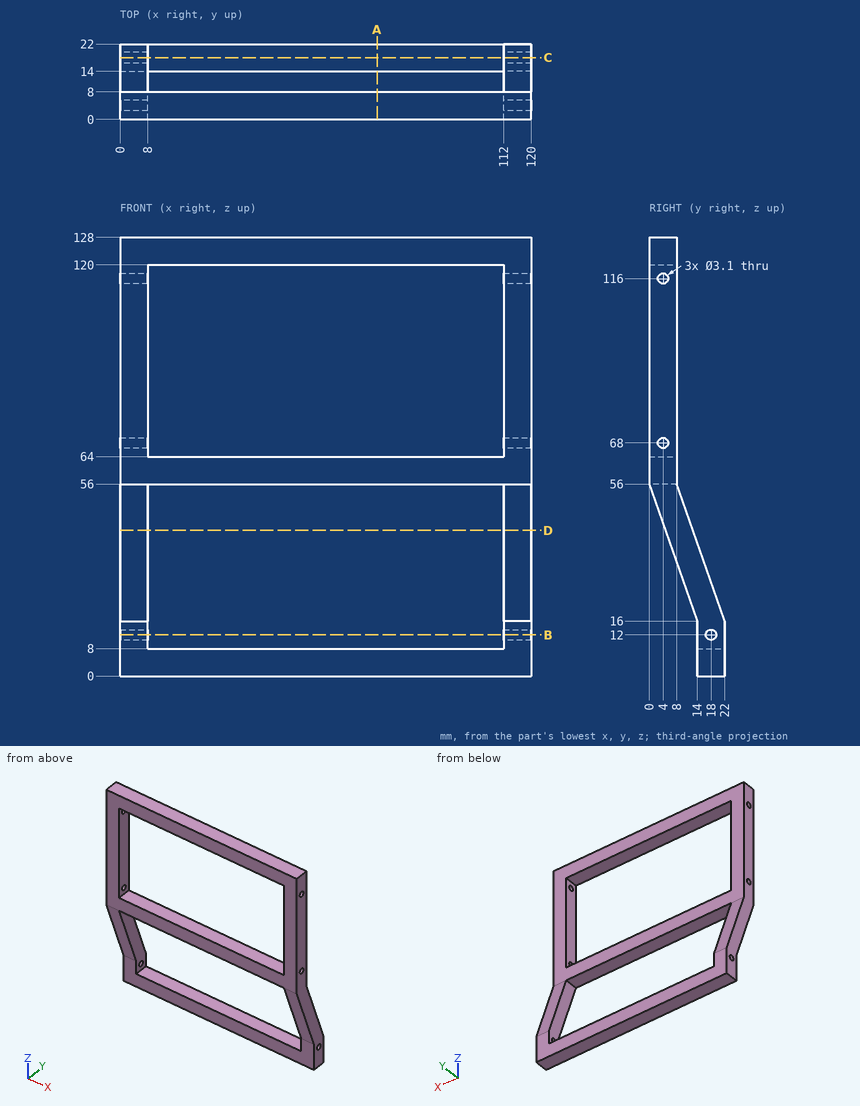
Could you check a few things on this drawing? It's one solid part, dimensions in mm from its lowest x, y, z. Round coordinates to 2 decimals unless told otherwise and drop trailing zeros. Write each loop counter-clockwise with the first axis right and the second up, starting at its lowest first coordinate (ties: lowest second). Pieces come first, ordered by that corner, then holes. Notation, with made-up numbers: (71, 13.5) -> (119, 13.5) arc R5 cw to (119, 17.5) -> close; hole circle Ø6 at (-21.75, 63). An arc over 180 degrees is marked (long way). Use a Markdown table: item, result.
1. If we section it at B-B (z = 12): List the corners of the cut face in (x, y) for me, then the cut area to 3 significant figures.
Answer key:
| item | result |
|---|---|
| outline | (0, 14) -> (8, 14) -> (8, 16.45) -> (0, 16.45) -> close; (0, 19.55) -> (8, 19.55) -> (8, 22) -> (0, 22) -> close; (112, 14) -> (120, 14) -> (120, 16.45) -> (112, 16.45) -> close; (112, 19.55) -> (120, 19.55) -> (120, 22) -> (112, 22) -> close |
| area | 78.4 mm^2 |
2. For pin 1 Ø8 at (x, z) = (65.5, 9.5) entering from -Y; pin 2 Ø4 at (x, y) = (71.5, 18.5) entering from +Z; pin 3 Ø1.9 at (y, z) = (4, 68) entering from -X; pin 4 Ø6.5 at (x, y) = (66, 6) entering from -Z, each with a flat end and sliding along its axis, tell me the tip position at first contact or that it passes through.
Answer key:
| item | result |
|---|---|
| pin 1 | stops at y = 14 |
| pin 2 | stops at z = 8 |
| pin 3 | passes through |
| pin 4 | stops at z = 56 |
3. Please list where these lines run through material, in increasing order: probe 1 along Y at (x, z) = (118, 116); probe 2 along X at (y, z) = (5.25, 117.5); probe 3 along Y at (x, z) = (5.75, 12).
Answer key:
| item | result |
|---|---|
| probe 1 | y = 0 to 2.45, 5.55 to 8 |
| probe 2 | x = 0 to 8, 112 to 120 |
| probe 3 | y = 14 to 16.45, 19.55 to 22 |
4. If we section it at D-D (z = 42.5): List the corners of the cut face in (x, y) for me (3 decimals), then the cut area to 3 significant figures.
Answer key:
| item | result |
|---|---|
| outline | (0, 4.725) -> (8, 4.725) -> (8, 12.725) -> (0, 12.725) -> close; (112, 4.725) -> (120, 4.725) -> (120, 12.725) -> (112, 12.725) -> close |
| area | 128 mm^2 |
5. If we section it at A-A (x = 75): List the corners of the cut face in (y, z) for me.
Answer key:
| item | result |
|---|---|
| outline | (0, 56) -> (8, 56) -> (8, 64) -> (0, 64) -> close; (0, 120) -> (8, 120) -> (8, 128) -> (0, 128) -> close; (14, 0) -> (22, 0) -> (22, 8) -> (14, 8) -> close |
6. If we section it at C-C (y = 18): List the corners of the cut face in (x, z) for me, then the cut area to 3 significant figures.
Answer key:
| item | result |
|---|---|
| outline | (0, 0) -> (120, 0) -> (120, 10.45) -> (112, 10.45) -> (112, 8) -> (8, 8) -> (8, 10.45) -> (0, 10.45) -> close; (0, 13.55) -> (8, 13.55) -> (8, 27.43) -> (0, 27.43) -> close; (112, 13.55) -> (120, 13.55) -> (120, 27.43) -> (112, 27.43) -> close |
| area | 1,220 mm^2 |
